The listing builds one solid part. Answer for the finished solid, in the listing's coordinates (mm). A direction names the side the tool comes from. Round coordinates to 2 decimals unless told otherwise and drop trailing zeros. Write each loop counter-clockwise with the first axis right and the second up, starting at its lowest first coordinate (ties: lowest second). Pieces come first, ordered by that corner, then holes. Notation, with made-up numbers: (-39.75, 69) - (2.25, 69) arc R14 ccw to (2.25, 95) - close; hole circle Ø1 at (24, 72). An arc over 180 degrees is marked (long way). Answer as CSV lines item,"result". Start each with the question number.
Item 1: Which of the six approach directions +Z, -Z, +X, -X, +Y, -Y give full straight-line access (tool end or side, diameter ignored) to faces 1 (the cylindrical face through (-72.743, -247.972, 19.761)), 2 (the flat face through (-63, -124, 0)), 3 (the flat face through (-62, -246, 49))?
Item 2: A cutting plane is placed at A-A on z = 46. Determine the outline of the cut face in (x, y).
Item 3: For a pull along X with two mould halves and no side action, classify faces 4 (the cylindrical face through (-38.564, -150.441, 2.284)), 5 (the flat face through (-75.385, -25.112, 50.256)), 6 (the cylindrical face through (-82.584, -243.062, 50.256)), 7 (the cylindrical face through (-76.7, -24.113, 2.284)) as pulls with the +X half, pulls with the -X half, needs draft (parallel to the pull), parting line crosses it, or undercut.
Item 4: A cutting plane is placed at C-C on z = 20. Determine the outline of the cut face in (x, y).
Item 5: A cutting plane is placed at B-B on y = -182. Determine the outline of the cut face in (x, z), and give its area (3 significant figures).
Item 6: Flat-ended cylindrical pins translate along their axes: pin 1 (8 mm diameter, centred on x = -67, z = 48.5, fed in from +Y); pin 2 (10 mm diameter, centred on x = -72, y = -84.5, fed in from +Z); pin 3 (10 mm diameter, centred on x = -48.5, z = 63, fed in from +Y); pin 4 (12 mm diameter, centred on x = -47.5, z = 27.5, fed in from -Y). Find the tip coordinate at first contact, or state that the pin passes through.
Item 7: Straight lines are drawn through the part: line 1 along X through (y, z) = (-101.5, 47); line 2 along Z through (x, y) = (-73, -28); line 3 along Y through (x, z) = (-47.5, 41.5). For each, find the intervals that lie inside material, in ascending order. Write a range as [from, to].
Autodesk Fusion 360 part; units mm, degrees
sketch "Sketch1" plane through (0, 0, 0) normal (0, 0, 1) x (1, 0, 0)
  line L0 (-36.1553, -250) -> (-89.3702, -250)
  line L1 (-89.3702, -250) -> (-89.3702, 17.3508)
  line L2 (-89.3702, 17.3508) -> (-36.1553, 17.3508)
  line L3 (-36.1553, 17.3508) -> (-36.1553, -250)
extrude "Extrude1" add sketch "Sketch1" along normal blind 95.2353
sketch "Sketch2" plane through (0, 0, 95.2353) normal (0, 0, 1) x (-1, 0, 0)
  line L0 (36.1553, -17.3508) -> (89.3702, -17.3508)
  line L1 (89.3702, -17.3508) -> (89.3702, 250)
  line L2 (89.3702, 250) -> (36.1553, 250)
  line L3 (36.1553, 250) -> (36.1553, -17.3508)
  line L4 (89.3702, 49.3912) -> (62.7627, -17.3508)
  line L5 (62.7627, -17.3508) -> (36.1553, 46.8639)
extrude "Extrude2" cut sketch "Sketch2" against normal blind 218.776 contours L0 L3 L5 | L0 L1 L4
fillet "Fillet1" radius 11.437 1 edges at (-62.7627, 17.3508, 47.6177)
fillet "Fillet2" radius 63.498 1 edges at (-89.3702, -49.3912, 47.6177)
fillet "Fillet3" radius 74.946 1 edges at (-36.1553, -46.8639, 47.6177)
fillet "Fillet4" radius 13.769 1 edges at (-89.3702, -250, 47.6177)
fillet "Fillet5" radius 13.342 1 edges at (-36.1553, -250, 47.6177)
shell "Shell1" thickness 4 removed faces 1 at (-53.8936, -178.2217, 95.2353)
fillet "Fillet8" radius 8.009 1 faces at (-53.8936, -178.2217, 0)
hole "Hole2" at (-62.3327, -250, 18.3944) direction (0, 1, 0) diameter 21 depth 30 tip angle 118
Geometry says:
1,face 1,"-Y"
1,face 2,"-Z, +X, -X, +Y, -Y"
1,face 3,"+Z"
2,outline,"(-89.37, -236.23) arc R13.77 ccw to (-75.6, -250) - (-49.5, -250) arc R13.34 ccw to (-36.16, -236.66) - (-36.16, -61.78) arc R74.95 ccw to (-41.86, -33.09) - (-51.99, -8.64) arc R11.44 ccw to (-73.18, -8.79) - (-84.86, -38.07) arc R63.5 ccw to (-89.37, -61.58) - close; hole (-85.37, -236.23) arc R9.77 ccw to (-75.6, -246) - (-49.5, -246) arc R9.34 ccw to (-40.16, -236.66) - (-40.16, -61.78) arc R70.95 ccw to (-45.56, -34.62) - (-55.69, -10.17) arc R7.44 ccw to (-69.47, -10.27) - (-81.14, -39.55) arc R59.5 ccw to (-85.37, -61.58) - close"
3,face 4,"pulls with the +X half"
3,face 5,"undercut"
3,face 6,"undercut"
3,face 7,"pulls with the -X half"
4,outline,"(-89.37, -236.23) arc R13.77 ccw to (-75.6, -250) - (-72.71, -250) - (-72.71, -246) - (-75.6, -246) arc R9.77 cw to (-85.37, -236.23) - (-85.37, -61.58) arc R59.5 cw to (-81.14, -39.55) - (-69.47, -10.27) arc R7.44 cw to (-55.69, -10.17) - (-45.56, -34.62) arc R70.95 cw to (-40.16, -61.78) - (-40.16, -236.66) arc R9.34 cw to (-49.5, -246) - (-51.96, -246) - (-51.96, -250) - (-49.5, -250) arc R13.34 ccw to (-36.16, -236.66) - (-36.16, -61.78) arc R74.95 ccw to (-41.86, -33.09) - (-51.99, -8.64) arc R11.44 ccw to (-73.18, -8.79) - (-84.86, -38.07) arc R63.5 ccw to (-89.37, -61.58) - close"
5,outline,"(-89.37, 8.01) arc R8.01 ccw to (-81.36, 0) - (-44.16, 0) arc R8.01 ccw to (-36.16, 8.01) - (-36.16, 95.24) - (-40.16, 95.24) - (-40.16, 4) - (-85.37, 4) - (-85.37, 95.24) - (-89.37, 95.24) - close"
5,area,"915 mm^2"
6,pin 1,"stops at y = -1.59"
6,pin 2,"stops at z = 4"
6,pin 3,"stops at y = -6.04"
6,pin 4,"stops at y = -250"
7,line 1,"x = [-89.37, -85.37], [-40.16, -36.16]"
7,line 2,"z = [0.03, 4]"
7,line 3,"y = [-249.85, -245.78], [-29.93, -19.48]"
